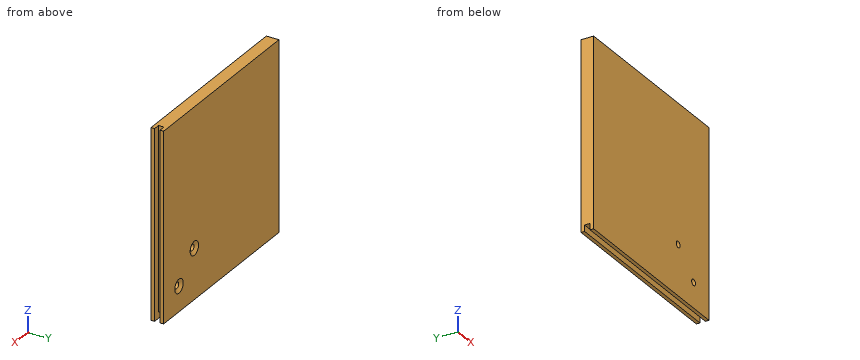
from build123d import *

# Parameters (mm, degrees)
SKETCH1_W               = 150
SKETCH1_H               = 150
BOSS_EXTRUDE1_DEPTH     = 10
CUT_EXTRUDE1_DEPTH      = 213.367605816
CUT_EXTRUDE1_DEPTH_BACK = 213.367605816
SKETCH2_W               = 5.1
SKETCH2_H               = 4.3
CUT_EXTRUDE2_DEPTH      = 209.796575642
CUT_EXTRUDE2_DEPTH_BACK = 209.796575642
SKETCH3_W               = 5
SKETCH3_H               = 4.3
CUT_EXTRUDE3_DEPTH      = 213.367605816
CUT_EXTRUDE3_DEPTH_BACK = 213.367605816
SKETCH4_R               = 2.5
CHAMFER1_SIZE           = 3
CHAMFER1_SIZE2          = 1.732050808


with BuildPart() as part:
    # Sketch1 → Boss-Extrude1 (new body)
    with BuildSketch(Plane(origin=(0, 0, 0), x_dir=(1, 0, 0), z_dir=(0, 1, 0))):
        with Locations((75, 75)):
            Rectangle(SKETCH1_W, SKETCH1_H)
    extrude(amount=BOSS_EXTRUDE1_DEPTH)

    # Sketch2 → Cut-Extrude1 (cut, two sides: drawn at the far end of the back side and taken through both)
    with BuildSketch(Plane.XY.offset(-CUT_EXTRUDE1_DEPTH_BACK)):
        with Locations((147.45, 5)):
            Rectangle(SKETCH2_W, SKETCH2_H)
    extrude(amount=CUT_EXTRUDE1_DEPTH + CUT_EXTRUDE1_DEPTH_BACK, mode=Mode.SUBTRACT)

    # Sketch3 → Cut-Extrude2 (cut, two sides: drawn at the far end of the back side and taken through both)
    with BuildSketch(Plane(origin=(144.9, 0, 0), x_dir=(0, 0, -1), z_dir=(1, 0, 0)).offset(-CUT_EXTRUDE2_DEPTH_BACK)):
        with Locations((147.5, 5)):
            Rectangle(SKETCH3_W, SKETCH3_H)
    extrude(amount=CUT_EXTRUDE2_DEPTH + CUT_EXTRUDE2_DEPTH_BACK, mode=Mode.SUBTRACT)

    # Sketch4 → Cut-Extrude3 (cut, two sides: drawn at the far end of the back side and taken through both)
    with BuildSketch(Plane(origin=(0, 10, 0), x_dir=(1, 0, 0), z_dir=(0, 1, 0)).offset(-CUT_EXTRUDE3_DEPTH_BACK)):
        with Locations(Location((130, 130, 0), (0, 0, 270))):
            Circle(SKETCH4_R)
        with Locations(Location((110, 110, 0), (0, 0, 270))):
            Circle(SKETCH4_R)
    extrude(amount=CUT_EXTRUDE3_DEPTH + CUT_EXTRUDE3_DEPTH_BACK, mode=Mode.SUBTRACT)

    # Chamfer1
    chamfer1_edges = [part.edges().sort_by_distance(p)[0] for p in [
        (130, 10, -132.5),
        (110, 10, -112.5),
    ]]
    chamfer1_side = [part.faces().sort_by_distance(p)[0] for p in [
        (74.921322866, 10, -74.921322866),
    ]]
    chamfer(chamfer1_edges, length=CHAMFER1_SIZE, length2=CHAMFER1_SIZE2, reference=chamfer1_side[0])


solid = part.part
Build history of the part. All positions in model axes, mm. Give positions to 0.01 mm unless a question says otherwise; leave off trailing zeros. Order: outer loops, then holes, each group sorted by start corner. A loop starts at its lowest first (then second) coordinate and runs counter-clockwise, first axis right, second up. Notation, with made-up numbers: M 45,85 L 80,85 A13 ccw 80,98 Z; hole C 13.25,6.5 d8. An arc over 180 degrees is marked long. Put each result on its own line as item: value.
Item 1: Cut at B-B on x = 130. Write the cut outline in (y, z).
Results are:
outline: M 0,-150 L 2.85,-150 L 2.85,-145 L 7.15,-145 L 7.15,-150 L 10,-150 L 10,-135.5 L 8.27,-132.5 L 0,-132.5 Z; M 0,-127.5 L 8.27,-127.5 L 10,-124.5 L 10,0 L 0,0 Z
Item 2: Wall check: probe 1 along X at (y, z) = (4, -110); probe 2 along Z at (x, y) = (130, 3.75); probe 3 along Z at (x, y) = (110, 4.25). Give the ranges that are in metal, low to high.
Results are:
probe 1: 0 to 107.5, 112.5 to 144.9
probe 2: -145 to -132.5, -127.5 to 0
probe 3: -145 to -112.5, -107.5 to 0
Item 3: Drop a flat-ended pin along its axis: pin 1 Ø4 at (x, y) = (102, 1.5) entering from +Z. Give the stop position or say it passes through.
Results are:
pin 1: z = 0
Item 4: Cut at A-A on z = -110. Write the cut outline in (x, y).
Results are:
outline: M 0,0 L 107.5,0 L 107.5,8.27 L 104.5,10 L 0,10 Z; M 112.5,0 L 150,0 L 150,2.85 L 144.9,2.85 L 144.9,7.15 L 150,7.15 L 150,10 L 115.5,10 L 112.5,8.27 Z
Item 5: Cut at C-C on y = 5.5. Write the cut outline in (x, z).
Results are:
outline: M 0,-145 L 144.9,-145 L 144.9,0 L 0,0 Z; hole C 110,-110 d5; hole C 130,-130 d5
